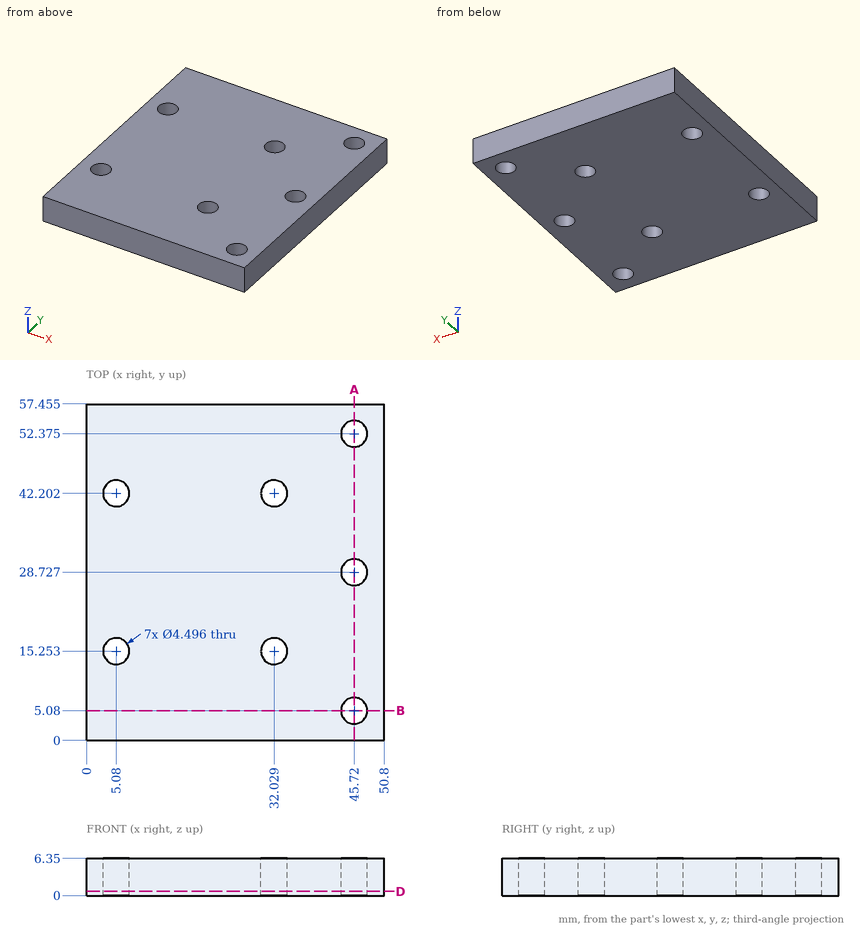
Can you work these out from the drawing? Everything is in mm from the part's minimum corner. Give positions to 0.01 mm unless a question says otherwise; leave off trailing zeros. Write each loop counter-clockwise with the first axis right and the second up, starting at its lowest first coordinate (ties: lowest second). Pieces come first, ordered by that corner, then holes. Notation, with made-up numbers: M 36,-38 L 91,-38 A12 cw 91,-29 Z; hole C -39.5,27 d4. An arc over 180 degrees is marked long. Answer in a Markdown table with one row per item. Add a question column.
Item 1: Imagine slicing it at D-D, the plane z = 0.75. Write out the boundary of the cut face in (x, y) (1 decimal), plus the area to 3 significant figures.
Item 2: Imagine slicing it at A-A, the plane x = 45.72. State how many separate pieces and enclosed holes the cut face has, plus the area to 3 significant figures.
Item 3: Imagine slicing it at B-B, the plane y = 5.08. Write out the boundary of the cut face in (x, z).
Item 4: Please list where these lines run through material, in increasing order: L1, parallel to Y at x = 5, z = 1 (1 decimal); L2, parallel to X at y = 42, z = 1; L3, parallel to Y at x = 45.72, z = 4.5 (1 decimal).
Evaluation:
| question | item | result |
|---|---|---|
| 1 | outline | M 0,0 L 50.8,0 L 50.8,57.5 L 0,57.5 Z; hole C 5.1,15.3 d4.5; hole C 5.1,42.2 d4.5; hole C 32,15.3 d4.5; hole C 32,42.2 d4.5; hole C 45.7,5.1 d4.5; hole C 45.7,28.7 d4.5; hole C 45.7,52.4 d4.5 |
| 1 | area | 2,810 mm² |
| 2 | separate pieces | 4 |
| 2 | enclosed holes | 0 |
| 2 | area | 279 mm² |
| 3 | outline | M 0,0 L 43.47,0 L 43.47,6.35 L 0,6.35 Z; M 47.97,0 L 50.8,0 L 50.8,6.35 L 47.97,6.35 Z |
| 4 | L1 | y = 0 to 13, 17.5 to 40, 44.4 to 57.5 |
| 4 | L2 | x = 0 to 2.84, 7.32 to 29.79, 34.27 to 50.8 |
| 4 | L3 | y = 0 to 2.8, 7.3 to 26.5, 31 to 50.1, 54.6 to 57.5 |
